Geometry: see drawing. Coordinates: mm, zero at the bounding-box minimum. Round coordinates to 2 decimals unless told otherwise and drop trailing zeros. Loops run counter-clockwise (first coordinate to the right, second up) from the corner with the lowest first, then second, coordinate; pieces in that order, holes last. Notation, with made-up numbers: (-26.5, 13.25) - (29.5, 13.25) arc R22 cw to (29.5, 43.25) - close; hole circle Ø6 at (-28, 60.25). An arc over 180 degrees is marked (long way). Write item = value, one per line. Start each with the question number.
Item 1: Section B-B (y = 5.75). Return loops of the section in (x, z), plus the area to 3 significant figures.
Item 2: Section C-C (x = 3). Return loops of the section in (y, z).
Item 3: Section D-D (x = 31.5). Return loops of the section in (y, z), plus the area to 3 significant figures.
Item 4: First-contact query: pin 1 (5 mm diameter, centred on x = 3, z = 8, fed in from -Y); pin 2 (4 mm diameter, centred on y = 5, z = 11.5, fed in from -X); pin 3 (3 mm diameter, centred on x = 39, z = 6, fed in from -Y); pin 4 (5 mm diameter, centred on y = 4, z = 18, fed in from +X). Flat tips, straight axial feed; report the tip coordinate or a pass-through.
Item 5: Draft query along X for the marked faces 1, 2 and 3. Return one class per face: pulls with the +X half, pulls with the -X half, needs draft (parallel to the pull), parting line crosses it, or undercut.
Item 6: Line query: line 1 (Z direction, x = 39.5, y = 0.5); line 2 (Y direction, x = 5.5, z = 7); line 3 (X direction, y = 2.75, z = 3.75). Output: solid intervals per line, ascending. Write a range as from..to.
Item 7: Section A-A (z = 20). Return loops of the section in (x, y), plus the area to 3 significant figures.
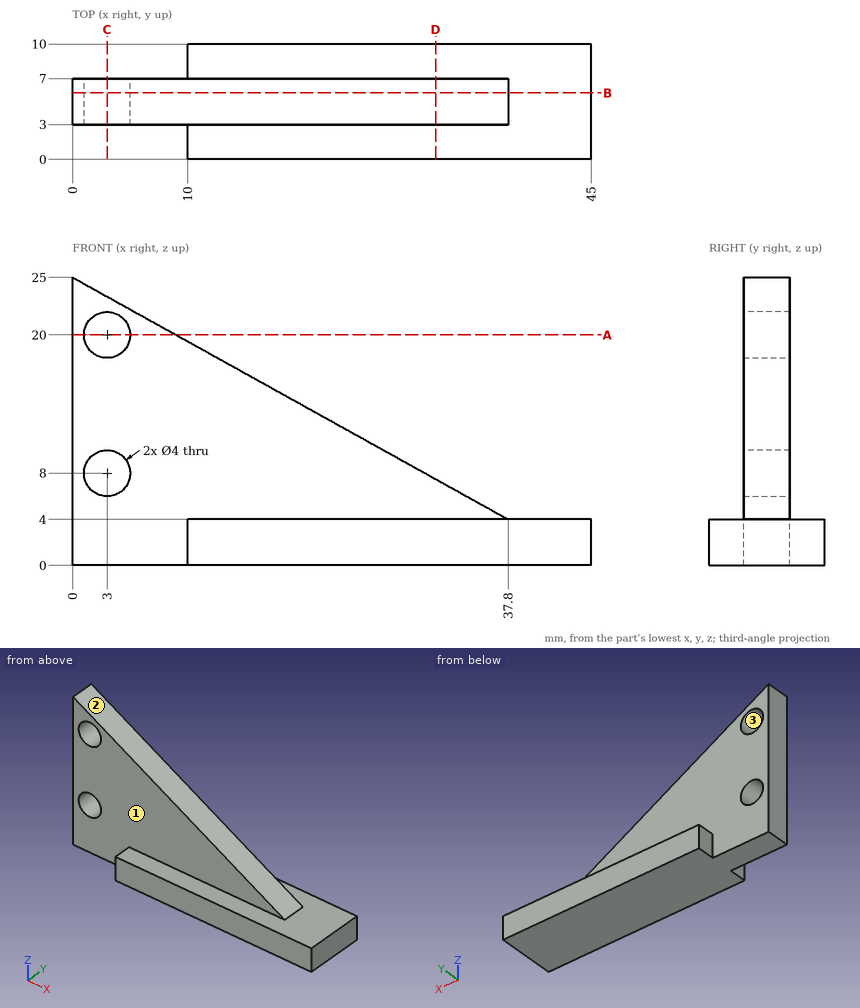
Taken from the geometry:
q1.outline = (0, 0) - (45, 0) - (45, 4) - (37.8, 4) - (0, 25) - close; hole circle Ø4 at (3, 8); hole circle Ø4 at (3, 20)
q1.area = 552 mm^2
q2.outline = (3, 0) - (7, 0) - (7, 6) - (3, 6) - close; (3, 10) - (7, 10) - (7, 18) - (3, 18) - close; (3, 22) - (7, 22) - (7, 23.33) - (3, 23.33) - close
q3.outline = (0, 0) - (10, 0) - (10, 4) - (7, 4) - (7, 7.5) - (3, 7.5) - (3, 4) - (0, 4) - close
q3.area = 54.0 mm^2
q4.pin_1 = 3
q4.pin_2 = 0
q4.pin_3 = through
q4.pin_4 = 17.1
q5.face_1 = needs draft
q5.face_2 = pulls with the +X half
q5.face_3 = undercut
q6.line_1 = 0..4
q6.line_2 = 3..7
q6.line_3 = 10..45
q7.outline = (0, 3) - (1, 3) - (1, 7) - (0, 7) - close; (5, 3) - (9, 3) - (9, 7) - (5, 7) - close
q7.area = 20.0 mm^2
